Geometry: final body of the model. Coordinates: model frame, mm. A direction names the side the tool comes from. Round coordinates to 2 decimals unless told otherwise and drop trailing zeros. Write each loop counter-clockwise with the first axis right and the second up, starting at its lowest first coordinate (ties: lowest second). Pieces come first, ordered by that corner, then holes. Notation, with made-up numbers: M 66,76 L 91,76 A17 cw 91,82 Z; hole C 28,71.25 d1. An arc over 180 degrees is marked long. Use one line per item in the form item = value. Start each with the question number.
Item 1: Section query A-A (y = 0). Return loops of the section in (x, z), and give its area (4 significant figures).
Item 2: Pull-direction query (X, two-part tool) for faces 1 (the flat face through (0, 30, -2)), 2 (the cylindrical face through (24.1, 24.14, -10.56)), 3 (the cylindrical face through (-29, 28, -2)); classes: pulls with the +X half, pulls with the -X half, needs draft (parallel to the pull), parting line crosses it, or undercut.
Item 3: Ray query, probe 1 along Y at (x, z) = (-22, -1.5); probe 2 along Y at (x, z) = (0, -3.6); probe 3 along Y at (x, z) = (20, -13). Return the intervals inside material, ascending.
Item 4: Pin query (flat end, axial travel): pin 1 Ø4 at (y, z) = (-4.5, -16.5) entering from -X; pin 2 Ø8 at (x, z) = (19, -14) entering from +Y; pin 3 Ø3 at (x, y) = (-23, 19) entering from -Z. Return the tip coordinate at first contact, or that it passes through.
Item 5: Reachability of faces 4 (the flat face through (12.562, -25.507, -10.437)), 5 (the flat face through (17, -25, -10)), 6 (the cylindrical face through (-26, 25, -9)), 7 (the flat face through (13, -26.5, -10.2)) from +Z, -Z, +X, -X, +Y, -Y: full face, straight path, thin tool, end or side. Return the list, or none.
Item 6: Section query C-C (z = -12). State how many separate pieces and enclosed holes the cut face has, and give its area (3 significant figures).
Autodesk Fusion 360 part; units mm, degrees
sketch "Common" plane through (0, 0, 0) normal (0, 0, 1) x (1, 0, 0)
  line L0 (30, -30) -> (-30, -30)
  line L1 (-30, -30) -> (-30, 30)
  line L2 (-30, 30) -> (30, 30)
  line L3 (30, 30) -> (30, -30)
  line L4 (30, -30) -> (-30, 30) construction
  line L5 (-30, -30) -> (30, 30) construction
  circle A0 centre (0, 0) radius 8
  circle A1 centre (0, 0) radius 10
  line L6 (-27, -27) -> (-27, 27)
  line L7 (-27, 27) -> (27, 27)
  line L8 (27, 27) -> (27, -27)
  line L9 (27, -27) -> (-27, -27)
  circle A2 centre (22, -22) radius 2
  circle A3 centre (22, 22) radius 2
  circle A4 centre (-22, 22) radius 2
  circle A5 centre (-22, -22) radius 2
  line L10 (25, -25) -> (-25, -25)
  line L11 (-25, -25) -> (-25, 25)
  line L12 (-25, 25) -> (25, 25)
  line L13 (25, 25) -> (25, -25)
  circle A6 centre (0, 0) radius 24.25
  dimension "d1" = 60
  dimension "d2" = 60
  dimension "d3" = 16
  dimension "d4" = 2
  dimension "d5" = 3
  dimension "d6" = 4
  dimension "d8" = 8
  dimension "d10" = 360
  dimension "d11" = 5
  dimension "d31" = 48.5
extrude "Extrude2" add sketch "Common" against normal blind 3 contours L0 L1 L2 L3 in component "Plug"
extrude "Extrude3" add sketch "Common" against normal blind 15 contours L6 L7 L8 L9 in component "Plug"
extrude "Extrude4" add sketch "Common" against normal blind 6 contours L10 L11 L12 L13 | A6 in component "Plug"
sketch "Flange cutout1" plane through (0, 0, 0) normal (0, 1, 0) x (1, 0, 0) in component "Plug"
  line L0 (0, 0) -> (0, 40) construction
  line L1 (0, 6) -> (10, 6)
  line L2 (10, 6) -> (25, 31.9808)
  line L3 (10, 6) -> (37, 6) construction
  line L4 (25, 31.9808) -> (0, 31.9808)
  line L5 (-25, 31.9808) -> (0, 31.9808)
  line L6 (0, 6) -> (-10, 6)
  line L7 (-10, 6) -> (-25, 31.9808)
  dimension "d90" = 40
  dimension "d91" = 10
  dimension "d92" = 6
  dimension "d93" = 30
  dimension "d94" = 60
extrude "Extrude6" cut sketch "Flange cutout1" along normal mid plane 100 in component "Plug"
sketch "Flange cutout2" plane through (0, 0, 0) normal (1, 0, 0) x (0, 1, 0) in component "Plug"
  line L0 (-25, -31.9808) -> (0, -31.9808)
  line L1 (0, -6) -> (10, -6)
  line L2 (-10, -6) -> (-25, -31.9808)
  line L3 (0, -6) -> (-10, -6)
  line L4 (-10, -6) -> (-37, -6) construction
  line L5 (0, 0) -> (0, -40) construction
  line L6 (10, -6) -> (25, -31.9808)
  line L7 (25, -31.9808) -> (0, -31.9808)
  point P0 (0.1488, 0.1515)
  dimension "d104" = 40
  dimension "d105" = 10
  dimension "d106" = 6
  dimension "d107" = 30
  dimension "d108" = 60
extrude "Extrude7" cut sketch "Flange cutout2" along normal mid plane 200 in component "Plug"
extrude "Extrude5" add sketch "Common" against normal blind 20 contours A1 in component "Plug"
fillet "Fillet1" radius 5 4 edges at (-30, -30, -1.5) (30, -30, -1.5) (30, 30, -1.5) (-30, 30, -1.5) in component "Plug"
fillet "Fillet1" radius 5 4 edges at (-27, 27, -9) (-27, -27, -9) (27, 27, -9) (27, -27, -9) in component "Plug"
fillet "Fillet1" radius 3 4 edges at (-25, 25, -10.5) (25, 25, -10.5) (-25, -25, -10.5) (25, -25, -10.5) in component "Plug"
extrude "Extrude8" cut sketch "Common" against normal blind 3 from surface at -3 contours A6 in component "Plug"
chamfer "Chamfer1" distance 1 angle 45 30 edges at (0, -30, 0) (-28.5355, -28.5355, 0) (-30, 0, 0) (-28.5355, 28.5355, 0) (0, 30, 0) (28.5355, 28.5355, 0) (30, 0, 0) (28.5355, -28.5355, 0) (27, -18.5981, -15) (25.5355, -25.5355, -15) (18.5981, -27, -15) (27, -12.5981, -10.5) (27, 12.5981, -10.5) (25.5355, 25.5355, -15) (27, 18.5981, -15) (18.5981, 27, -15) (-18.5981, 27, -15) (-25.5355, 25.5355, -15) (-27, 18.5981, -15) (-18.5981, -27, -15) (-25.5355, -25.5355, -15) (-27, -18.5981, -15) (-12.5981, -27, -10.5) (-12.5981, 27, -10.5) (12.5981, 27, -10.5) (12.5981, -27, -10.5) (-27, -12.5981, -10.5) (-27, 12.5981, -10.5) (-7.4586, -2.8929, -20) (-22.6089, -8.7692, -6) in component "Plug"
component "Plug" placed x (1, 0, 0) y (0, 1, 0) z (0, 0, 1) at (0, 0, 0)
Working result:
q1.outline = M -30,-3 L -27,-3 L -27,-6 L -25.25,-6 L -24.25,-5 L -24.25,-3 L -10,-3 L -10,-20 L -9,-20 L -8,-19 L -8,0 L -29,0 L -30,-1 Z; M 8,-19 L 9,-20 L 10,-20 L 10,-3 L 24.25,-3 L 24.25,-5 L 25.25,-6 L 27,-6 L 27,-3 L 30,-3 L 30,-1 L 29,0 L 8,0 Z
q1.area = 213.5 mm²
q2.face_1 = needs draft
q2.face_2 = undercut
q2.face_3 = pulls with the -X half
q3.probe_1 = -30 to -24, -20 to 20, 24 to 30
q3.probe_2 = -27 to -24.25, -10 to -8, 8 to 10, 24.25 to 27
q3.probe_3 = -27 to -25, 25 to 27
q4.pin_1 = -9.68
q4.pin_2 = 27
q4.pin_3 = -6
q5.face_4 = -Z, +Y, -Y
q5.face_5 = -Z
q5.face_6 = -Z, -X, +Y
q5.face_7 = -Z, -Y
q6.separate_pieces = 5
q6.enclosed_holes = 1
q6.area = 295 mm²
